```python
from build123d import *

# Parameters (mm, degrees)
F1_DEPTH = 2.54
F3_DEPTH = 25.4


with BuildPart() as f1:
    # F0 (on Right) → F1 (new body, symmetric)
    with BuildSketch(Plane.YZ):
        with BuildLine():
            Line((-43.832254, 7.411134), (-58.425114, 7.411134))
            Line((-58.425114, 7.411134), (-56.307647, -5.898658))
            Line((-56.307647, -5.898658), (-44.975612, 0))
            Line((-44.975612, 0), (-40.973853, -1.664879))
            ThreePointArc((-40.973853, -1.664879), (-36.253593, 5.184437), (-28.015766, 6.338645))
            Line((-28.015766, 6.338645), (-14.066866, 6.648439))
            Line((-14.066866, 6.648439), (-12.56959, 5.472009))
            ThreePointArc((-12.56959, 5.472009), (-9.908052, 6.78319), (-7.008282, 7.411134))
            Line((-7.008282, 7.411134), (8.071418, 8.787404))
            Line((8.071418, 8.787404), (8.071418, 11.247213))
            Line((8.071418, 11.247213), (-13.639072, 11.247213))
            Line((-13.639072, 11.247213), (-13.639072, 10.202761))
            Line((-13.639072, 10.202761), (-37.399668, 10.202761))
            Line((-37.399668, 10.202761), (-40.973853, 7.411134))
            ThreePointArc((-40.973853, 7.411134), (-42.403053, 7.069715), (-43.832254, 7.411134))
        make_face()
    extrude(amount=F1_DEPTH, both=True)

    # F2 (on face) → F3 (cut)
    with BuildSketch(Plane.XY.offset(10.202761)):
        Polygon((-1.27, -15.166366), (-1.27, -25.51937), (-1.27, -35.916388), (1.27, -35.916388), (1.27, -25.51937), (1.27, -15.166366), align=None)
    extrude(amount=-F3_DEPTH, mode=Mode.SUBTRACT)


solid = f1.part
```
For this review, take the finished solid that the model builds, in its own axes (mm). A direction names the side the tool comes from. Round coordinates to 2 decimals unless told otherwise and drop trailing zeros. Write each loop counter-clockwise with the first axis right and the second up, starting at its lowest first coordinate (ties: lowest second). Pieces come first, ordered by that corner, then holes. Notation, with made-up numbers: (64.5, 44.25) - (93.5, 44.25) arc R25 ccw to (93.5, 65.25) - close; hole circle Ø2 at (-36, 60.5). An arc over 180 degrees is marked (long way). Write each question's results on one line, items separated by ' | '.
Item 1: To check wall thickness, follow line 1 along X through (y, z) = (-20.5, 10); line 2 along Z through (x, y) = (-1.8, -45); line 3 along Y through (x, z) = (2.05, 5.75). State the ranges of each line that lie inside material, in increasing order. Write a range as from..to.
Calculated:
line 1: x = -2.54..-1.27, 1.27..2.54 | line 2: z = -0.01..7.41 | line 3: y = -58.16..-35.21, -12.92..-12.12
Item 2: Draft analysis for pull direction Y (two halves, no side actions). For faces 1 (the face through (0.04, -42.38, 7.07)), 2 (the face through (0, -3, 11.247)), 3 (the face through (0, 8.071, 10)), state which applies: pulls with the +Y half, pulls with the -Y half, needs draft (parallel to the pull), parting line crosses it, or undercut.
Calculated:
face 1: undercut | face 2: needs draft | face 3: pulls with the +Y half
Item 3: Take a section at B-B on y = -30.5. State the section outline as (x, z) points.
Calculated:
outline: (-2.54, 6.72) - (-1.27, 6.72) - (-1.27, 10.2) - (-2.54, 10.2) - close; (1.27, 6.72) - (2.54, 6.72) - (2.54, 10.2) - (1.27, 10.2) - close
Item 4: Take a section at A-A on x = 0. State the section outline as (y, z) points, then the cut area to 3 significant figures.
Calculated:
outline: (-58.43, 7.41) - (-56.31, -5.9) - (-44.98, 0) - (-40.97, -1.66) arc R10.34 cw to (-35.92, 5.38) - (-35.92, 10.2) - (-37.4, 10.2) - (-40.97, 7.41) arc R3.16 cw to (-43.83, 7.41) - close; (-15.17, 6.62) - (-14.07, 6.65) - (-12.57, 5.47) arc R12.17 cw to (-7.01, 7.41) - (8.07, 8.79) - (8.07, 11.25) - (-13.64, 11.25) - (-13.64, 10.2) - (-15.17, 10.2) - close | area: 279 mm^2
Item 5: For faces 4 (the face through (2, -25, 10.203)), 5 (the face through (0.04, -50.72, -2.99)), 6 (the face through (-1.27, -25, 8)), list the 3-axis set-ups (+Z, -Z, +X, -X, +Y, -Y) from which the entire face can be reached by the end or side of a thin tool; tool diameter is ignored.
Calculated:
face 4: +Z, +X, -X, -Y | face 5: -Z, +X, -X | face 6: +Z, -Z
Item 6: Take a section at C-C on z = -4. State the section outline as (x, y) points.
Calculated:
outline: (-2.54, -56.61) - (2.54, -56.61) - (2.54, -52.66) - (-2.54, -52.66) - close
Item 7: Take a section at D-D on y = 1. State the section outline as (x, z) points, then the cut area to 3 significant figures.
Calculated:
outline: (-2.54, 8.14) - (2.54, 8.14) - (2.54, 11.25) - (-2.54, 11.25) - close | area: 15.8 mm^2
Item 8: For pin 1 (0.8 mm diameter, centred on x = 0.5, z = 8.5, fed in from -Y); pin 2 (3 mm diameter, centred on x = 1, z = -3.5, fed in from +Y); pin 3 (1 mm diameter, centred on x = 1, z = 1, fed in from +Y), all flat-tipped, find the tip position at first contact; note any pin that passes through.
Calculated:
pin 1: stops at y = -40.09 | pin 2: stops at y = -48.82 | pin 3: stops at y = -39.81
